Verification items for the finished model (mm, model axes). A direction names the side the tool comes from. Round coordinates to 2 decimals unless told otherwise and drop trailing zeros. Write each loop counter-clockwise with the first axis right and the second up, starting at its lowest first coordinate (ties: lowest second). Pieces come first, ordered by that corner, then holes. Notation, with made-up numbers: (53.5, -8) -> (69.5, -8) arc R25 ccw to (69.5, 22) -> close; hole circle Ø2 at (-25.75, 49.5). An arc over 180 degrees is marked (long way). Use CSV: the item, a comma, the result in double quotes.
```python
from build123d import *

# Parameters (mm, degrees)
SKETCH1_W             = 35.5
SKETCH1_H             = 22
BOSS_EXTRUDE1_DEPTH   = 42
CUT_EXTRUDE1_DEPTH    = 60.230482017
SKETCH3_W             = 3
SKETCH3_H             = 3
CUT_EXTRUDE2_DEPTH    = 28
SKETCH4_W             = 29.5
SKETCH4_H             = 10
CUT_EXTRUDE3_DEPTH    = 19
F_2_5MM_DOWEL_HOLE1_D = 2.5
F_2_5MM_DOWEL_HOLE2_D = 2.5
FILLET1_R             = 0.5


with BuildPart() as part:
    # Sketch1 → Boss-Extrude1 (new body)
    with BuildSketch(Plane(origin=(0, 0, 0), x_dir=(1, 0, 0), z_dir=(0, 1, 0))):
        with Locations((17.75, 11)):
            Rectangle(SKETCH1_W, SKETCH1_H)
    extrude(amount=BOSS_EXTRUDE1_DEPTH)

    # Sketch2 → Cut-Extrude1 (cut, through all)
    with BuildSketch(Plane(origin=(35.5, 0, 0), x_dir=(0, 0, -1), z_dir=(1, 0, 0))):
        Polygon((0, 6), (19, 14), (19, 42), (0, 42), align=None)
    extrude(amount=-CUT_EXTRUDE1_DEPTH, mode=Mode.SUBTRACT)

    # Sketch3 → Cut-Extrude2 (cut)
    with BuildSketch(Plane(origin=(0, 42, 0), x_dir=(1, 0, 0), z_dir=(0, 1, 0))):
        with Locations((1.5, 20.5)):
            Rectangle(SKETCH3_W, SKETCH3_H)
        with Locations((34, 20.5)):
            Rectangle(SKETCH3_W, SKETCH3_H)
    extrude(amount=-CUT_EXTRUDE2_DEPTH, mode=Mode.SUBTRACT)

    # Sketch4 → Cut-Extrude3 (cut)
    with BuildSketch(Plane.XY):
        with Locations((17.75, 11)):
            Rectangle(SKETCH4_W, SKETCH4_H)
    extrude(amount=-CUT_EXTRUDE3_DEPTH, mode=Mode.SUBTRACT)

    # Sketch6 → Hole1 (revolve, cut)
    with BuildSketch(Plane(origin=(17.75, 0, -7.75), x_dir=(0, 0, -1), z_dir=(1, 0, 0))):
        Polygon((0, 0), (0, 42), (4.5, 42), (4.5, 5), (2.5, 5), (2.5, 0), align=None)
    revolve(axis=Axis((17.75, 110, -7.75), (0, -1, 0)), mode=Mode.SUBTRACT)

    # Ø2.5mm Dowel Hole1 (through all)
    with Locations(Plane(origin=(0, 0, 0), x_dir=(-1, 0, 0), z_dir=(0, -1, 0))):
        with Locations((-22.25, 7.75), (-13.25, 7.75)):
            Hole(F_2_5MM_DOWEL_HOLE1_D / 2)

    # Ø2.5mm Dowel Hole2 (through all)
    with Locations(Plane(origin=(0, 0, -22), x_dir=(-1, 0, 0), z_dir=(0, 0, -1))):
        with Locations((-10, 17.5), (-25.5, 17.5), (-25.5, 34.5), (-10, 34.5)):
            Hole(F_2_5MM_DOWEL_HOLE2_D / 2)

    # Fillet1
    # the kernel refuses this fillet: 0.5 mm, written as the material it takes off along each edge
    with BuildSketch(Plane(origin=(35.5, -1.25, 0), x_dir=(-1, 0, 0), z_dir=(0, 1, 0))) as fillet1_piece_1:
        with BuildLine():
            CenterArc((FILLET1_R, -FILLET1_R), FILLET1_R, 90, 90)
            Line((0, -FILLET1_R), (0, 0))
            Line((0, 0), (FILLET1_R, 0))
        make_face()
    extrude(amount=8.5, mode=Mode.SUBTRACT)
    with BuildSketch(Plane(origin=(0, -1.25, 0), x_dir=(1, 0, 0), z_dir=(0, 1, 0))) as fillet1_piece_2:
        with BuildLine():
            CenterArc((FILLET1_R, FILLET1_R), FILLET1_R, 180, 90)
            Line((0, FILLET1_R), (0, 0))
            Line((0, 0), (FILLET1_R, 0))
        make_face()
    extrude(amount=8.5, mode=Mode.SUBTRACT)
    with BuildSketch(Plane(origin=(0, -1.25, -22), x_dir=(0, 0, 1), z_dir=(0, 1, 0))) as fillet1_piece_3:
        with BuildLine():
            CenterArc((FILLET1_R, FILLET1_R), FILLET1_R, 180, 90)
            Line((0, FILLET1_R), (0, 0))
            Line((0, 0), (FILLET1_R, 0))
        make_face()
    extrude(amount=16.5, mode=Mode.SUBTRACT)
    with BuildSketch(Plane(origin=(35.5, -1.25, -22), x_dir=(0, 0, 1), z_dir=(0, 1, 0))) as fillet1_piece_4:
        with BuildLine():
            CenterArc((FILLET1_R, -FILLET1_R), FILLET1_R, 90, 90)
            Line((0, -FILLET1_R), (0, 0))
            Line((0, 0), (FILLET1_R, 0))
        make_face()
    extrude(amount=16.5, mode=Mode.SUBTRACT)
    with BuildSketch(Plane(origin=(3, 43.25, -22), x_dir=(1, 0, 0), z_dir=(0, -1, 0))) as fillet1_piece_5:
        with BuildLine():
            CenterArc((FILLET1_R, FILLET1_R), FILLET1_R, 180, 90)
            Line((0, FILLET1_R), (0, 0))
            Line((0, 0), (FILLET1_R, 0))
        make_face()
    extrude(amount=29.25, mode=Mode.SUBTRACT)
    with BuildSketch(Plane(origin=(3, 43.25, -19), x_dir=(1, 0, 0), z_dir=(0, -1, 0)), Plane(origin=(32.5, 14, -19), x_dir=(-1, 0, 0), z_dir=(0, 1, 0)), Plane(origin=(32.5, 43.25, -22), x_dir=(-1, 0, 0), z_dir=(0, -1, 0))) as fillet1_piece_6:
        with BuildLine():
            CenterArc((FILLET1_R, -FILLET1_R), FILLET1_R, 90, 90)
            Line((0, -FILLET1_R), (0, 0))
            Line((0, 0), (FILLET1_R, 0))
        make_face()
    extrude(amount=29.25, mode=Mode.SUBTRACT)


solid = part.part
```
Q1. Access from +Z, -Z, +X, -X, +Y, -Y to the whole of each face (thin tool, end or side, straight path). Record for faces 4 (the flat face through (14, 6, -11)), 5 (the flat face through (3, 28, -20)), 6 (the flat face through (18, 21, -22)).
Filled in:
face 4,"+Z, +Y"
face 5,"+Z, -Z, -X, +Y"
face 6,"-Z, +X, -X, +Y, -Y"
Q2. Mould release check, pull along Z, two halves, no side actions. Record for faces 1 (the flat face through (34.021, 9.944, -9.367)), 2 (the cylindrical face through (8.75, 17.55, -20.48)), 3 (the flat face through (16, 5, -10)): released by +Z, released by -Z, zero draft, split by the parting line, or undercut.
Filled in:
face 1,"released by +Z"
face 2,"zero draft"
face 3,"undercut"
Q3. Section check D-D (x = 29). Record the cut outline in (y, z), plus the area to 3 significant figures.
Filled in:
outline,"(0, -22) -> (42, -22) -> (42, -19) -> (6, -19) -> (6, 0) -> (0, 0) -> close"
area,"240 mm²"
Q4. Section check A-A (y = 17.5). Record the cut outline in (x, z).
Filled in:
outline,"(3, -21.5) arc R0.5 ccw to (3.5, -22) -> (8.75, -22) -> (8.75, -19) -> (3.5, -19) arc R0.5 ccw to (3, -19.5) -> close; (11.25, -22) -> (24.25, -22) -> (24.25, -19) -> (11.25, -19) -> close; (26.75, -22) -> (32, -22) arc R0.5 ccw to (32.5, -21.5) -> (32.5, -19.5) arc R0.5 ccw to (32, -19) -> (26.75, -19) -> close"
Q5. Section check B-B (x = 17.75). Record the cut outline in (y, z).
Filled in:
outline,"(0, -22) -> (42, -22) -> (42, -19) -> (6, -19) -> (6, -12.25) -> (5, -12.25) -> (5, -10.25) -> (0, -10.25) -> close; (0, -5.25) -> (5, -5.25) -> (5, -3.25) -> (6, -3.25) -> (6, 0) -> (0, 0) -> close"
Q6. Material ranges on L1, parallel to Y at x = 10, z = -20.5; L2, parallel to X at y = 4.05, z = -7.75; L3, parallel to X at y = 10.5, z = -14.25, recorded low to high.
Filled in:
L1,"0 to 16.25, 18.75 to 33.25, 35.75 to 42"
L2,"0 to 12, 14.5 to 15.25, 20.25 to 21, 23.5 to 35.5"
L3,"0 to 3, 32.5 to 35.5"
Q7. Go/stop test with flat-tipped pins: P1, Ø1.6, axis at y = 31, z = -20, coming from the +X side; P2, Ø0.9, axis at x = 33.5, z = -21, coming from the +Y side; P3, Ø4, axis at x = 13.25, z = -7.75, coming from the +Y side; P4, Ø2, axis at x = 25.5, y = 17.5, coming from the -Z side. Record where each tip stops, or that it passes through.
Filled in:
P1,"x = 32.5"
P2,"y = 14"
P3,"y = 6"
P4,"through"
Q8. Section check C-C (z = -6). Record the cut outline in (x, y), plus the area to 3 significant figures.
Filled in:
outline,"(0, 0) -> (15.96, 0) -> (15.96, 5) -> (13.6, 5) -> (13.6, 6) -> (3, 6) -> (3, 8.53) -> (0, 8.53) -> close; (19.54, 0) -> (35.5, 0) -> (35.5, 8.53) -> (32.5, 8.53) -> (32.5, 6) -> (21.9, 6) -> (21.9, 5) -> (19.54, 5) -> close"
area,"202 mm²"
